The listing builds one solid part. Answer for the finished solid, in the listing's coordinates (mm). A direction names the side the tool comes from. Coordinates: 2 decimals unless noted, no trailing zeros. Loops run counter-clockwise (first coordinate to the right, second up) from the corner with the lowest first, then second, coordinate; pieces in that order, holes last. Notation, with made-up numbers: M 1,38 L 42,38 A19 cw 42,64 Z; hole C -8.75,-30 d11. An arc over 180 degrees is marked long. Return JSON: item names as keys, results as strings. Group by question number.
1. Section D-D (z = -0.25) is taken. Write down the section's boundary in (x, y).
2. Section C-C (z = -4.25) is taken. Write down the section's boundary in (x, y), then the cut area to 3 significant figures.
3. Section A-A (y = 0) is taken. Write down the section's boundary in (x, z).
4. Given P1, Ø4, axis at y = -4.5, z = -4, coming from the -X side; P2, Ø3, axis at x = -5, y = -3, coming from the -Z side; P3, Ø3, axis at y = 2.5, z = -3.5, coming from the +X side, each flat-ended and moving along its own axis, determine where each tip first touches the part or whether it passes through.
5. Which of the six approach directions +Z, -Z, +X, -X, +Y, -Y give full straight-line access (tool end or side, diameter ignored) to faces 1 (the face through (-2, -1, -3.7)), 2 (the face through (0, 0, 2))?
6. Straight lines are drawn through the part: L1, parallel to Z at x = 3, y = 4.25; L2, parallel to Y at x = 0, z = -2.75; L3, parallel to Z at x = 1.5, y = -2. For each, find the intervals that lie inside material, in ascending order. Write a range as from..to.
```python
from build123d import *

# Parameters (mm, degrees)
F0_R     = 7
F0_R_2   = 4
F0_R_3   = 2
F1_DEPTH = 2
F2_SIZE  = 1
F3_DEPTH = 7.3
F4_DEPTH = 3.7


with BuildPart() as f1:
    # F0 (on Top) → F1 (new body)
    with BuildSketch(Plane.XY):
        Circle(F0_R)
        Circle(F0_R_2, mode=Mode.SUBTRACT)
        Circle(F0_R_2)
        Circle(F0_R_3, mode=Mode.SUBTRACT)
        Circle(F0_R_3)
    extrude(amount=F1_DEPTH)

    # F2
    f2_edges = [f1.edges().sort_by_distance(p)[0] for p in [
        (-7, 0, 2),
    ]]
    chamfer(f2_edges, length=F2_SIZE)

    # F0 (on Top) → F3 (join)
    with BuildSketch(Plane.XY):
        Circle(F0_R_3)
    extrude(amount=-F3_DEPTH)

    # F0 (on Top) → F4 (join)
    with BuildSketch(Plane.XY):
        Circle(F0_R_2)
        Circle(F0_R_3, mode=Mode.SUBTRACT)
    extrude(amount=-F4_DEPTH)


solid = f1.part
```
Worked out:
{
 "1": {"outline": "C 0,0 d8"},
 "2": {"outline": "C 0,0 d4", "area": "12.6 mm^2"},
 "3": {"outline": "M -7,0 L -4,0 L -4,-3.7 L -2,-3.7 L -2,-7.3 L 2,-7.3 L 2,-3.7 L 4,-3.7 L 4,0 L 7,0 L 7,1 L 6,2 L -6,2 L -7,1 Z"},
 "4": {"P1": "x = -3.1", "P2": "z = 0", "P3": "x = 3.87"},
 "5": {"face 1": "-Z", "face 2": "+Z, +X, -X, +Y, -Y"},
 "6": {"L1": "0..2", "L2": "-4..4", "L3": "-3.7..2"}
}
